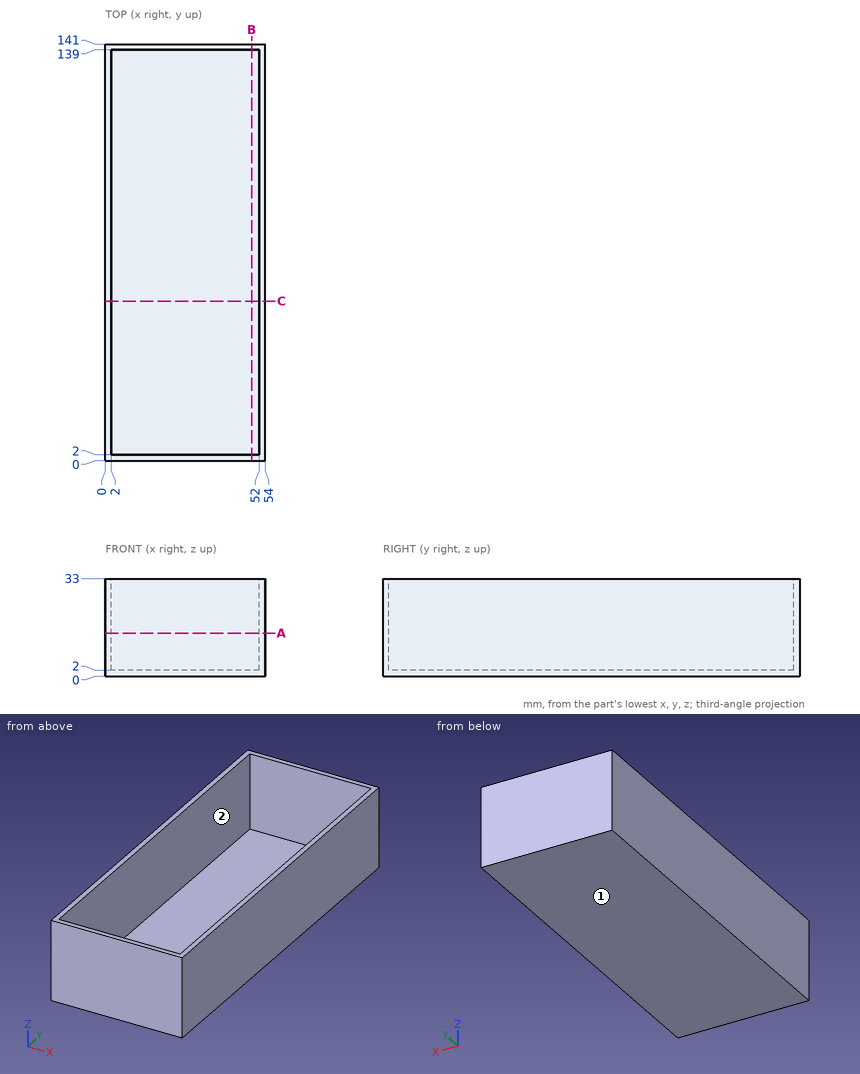
Here's the drawing with two shaded views (mm, measured from the low corner). I have some questions. A direction names the side the tool comes from. Round coordinates to 2 decimals unless told otherwise and drop trailing zeros. Loops run counter-clockwise (first coordinate to the right, second up) from the corner with the lowest first, then second, coordinate; pieces in that order, holes last. Notation, with made-up numbers: (-11.5, -18) - (5.5, -18) arc R20 ccw to (5.5, 18) - close; hole circle Ø10 at (-34, -16). An arc over 180 degrees is marked (long way). Use CSV: the item, a comma, the result in double quotes. Start each with the question number.
1) For pin 1 Ø3 at (x, y) = (14.5, 119.5) entering from +Z, with a flat end and sliding along its axis, tell me the tip position at first contact or that it passes through.
2) If we section it at C-C on y = 54: Write out the boundary of the cut face in (x, z), plus the area to 3 significant figures.
3) For the marked faces 1 and 2, which set-ups out of +Z, -Z, +X, -X, +Y, -Y let a thin tool reach every point of the face, with its end or its side?
4) If we section it at B-B on x = 49.5: Write out the boundary of the cut face in (y, z), plus the area to 3 significant figures.
5) Please list where these lines run through material, in increasing order: probe 1 along X at (y, z) = (70, 23); probe 2 along Y at (x, z) = (14, 12.5); probe 3 along Z at (x, y) = (34, 66). Write a range as [from, to].
6) If we section it at A-A on z = 14.5: Write out the boundary of the cut face in (x, y), plus the area to 3 significant figures.
Geometry results:
1,pin 1,"stops at z = 2"
2,outline,"(0, 0) - (54, 0) - (54, 33) - (52, 33) - (52, 2) - (2, 2) - (2, 33) - (0, 33) - close"
2,area,"232 mm2"
3,face 1,"-Z, +X, -X, +Y, -Y"
3,face 2,"+Z"
4,outline,"(0, 0) - (141, 0) - (141, 33) - (139, 33) - (139, 2) - (2, 2) - (2, 33) - (0, 33) - close"
4,area,"406 mm2"
5,probe 1,"x = [0, 2], [52, 54]"
5,probe 2,"y = [0, 2], [139, 141]"
5,probe 3,"z = [0, 2]"
6,outline,"(0, 0) - (54, 0) - (54, 141) - (0, 141) - close; hole (2, 2) - (52, 2) - (52, 139) - (2, 139) - close"
6,area,"764 mm2"
